```python
from build123d import *

# Parameters (mm, degrees)
EXTRUDE_1_DEPTH     = 280
SKETCH_2_R          = 2.2
CUT_EXTRUDE_1_DEPTH = 280
SKETCH_3_R          = 2.2
CUT_EXTRUDE_2_DEPTH = 20
CUT_EXTRUDE_3_DEPTH = 59
EXTRUDE_3_DEPTH     = 20
SKETCH_6_W          = 4.4
SKETCH_6_H          = 18
CUT_EXTRUDE_4_DEPTH = 20


with BuildPart() as part:
    # 草图1 → 凸台-拉伸1 (new body)
    with BuildSketch(Plane(origin=(0, 0, 0), x_dir=(1, 0, 0), z_dir=(0, 1, 0))):
        Polygon((10, 0), (10, 10), (0, 10), (-10, 10), (-10, 0), (-10, -10), (0, -10), (10, -10), align=None)
        Polygon((9, 0), (9, 9), (0, 9), (-9, 9), (-9, 0), (-9, -9), (0, -9), (9, -9), align=None, mode=Mode.SUBTRACT)
    extrude(amount=-EXTRUDE_1_DEPTH)

    # 草图2 → 切除-拉伸1 (cut)
    with BuildSketch(Plane.XY.offset(10)):
        with Locations(Location((0, -40, 0), (0, 0, 180))):
            Circle(SKETCH_2_R)
        with Locations(Location((0, -80, 0), (0, 0, 180))):
            Circle(SKETCH_2_R)
        with Locations(Location((0, -120, 0), (0, 0, 180))):
            Circle(SKETCH_2_R)
        with Locations(Location((0, -180, 0), (0, 0, 180))):
            Circle(SKETCH_2_R)
        with Locations(Location((0, -220, 0), (0, 0, 180))):
            Circle(SKETCH_2_R)
        with Locations(Location((0, -260, 0), (0, 0, 180))):
            Circle(SKETCH_2_R)
    extrude(amount=-CUT_EXTRUDE_1_DEPTH, mode=Mode.SUBTRACT)

    # 草图3 → 切除-拉伸2 (cut)
    with BuildSketch(Plane(origin=(10, 0, 0), x_dir=(0, 0, -1), z_dir=(1, 0, 0))):
        with Locations((0, -60)):
            Circle(SKETCH_3_R)
        with Locations((0, -100)):
            Circle(SKETCH_3_R)
        with Locations((0, -150)):
            Circle(SKETCH_3_R)
        with Locations((0, -200)):
            Circle(SKETCH_3_R)
        with Locations((0, -240)):
            Circle(SKETCH_3_R)
    extrude(amount=-CUT_EXTRUDE_2_DEPTH, mode=Mode.SUBTRACT)

    # 草图4 → 切除-拉伸3 (cut)
    with BuildSketch(Plane.XY.offset(10)):
        Polygon((0, -220), (10, -220), (10, 0), (-10, 0), (-10, -220), align=None)
    extrude(amount=-CUT_EXTRUDE_3_DEPTH, mode=Mode.SUBTRACT)

    # 草图5 → 凸台-拉伸3 (add)
    with BuildSketch(Plane.XY.offset(10)):
        with BuildLine():
            Line((-2.2, -220), (2.2, -220))
            ThreePointArc((2.2, -220), (0, -222.2), (-2.2, -220))
        make_face()
    extrude(amount=-EXTRUDE_3_DEPTH)

    # 草图6 → 切除-拉伸4 (cut)
    with BuildSketch(Plane(origin=(0, -220, 0), x_dir=(1, 0, 0), z_dir=(0, 1, 0))):
        Rectangle(SKETCH_6_W, SKETCH_6_H)
    extrude(amount=-CUT_EXTRUDE_4_DEPTH, mode=Mode.SUBTRACT)


solid = part.part
```
Geometry check sheet. Reference: the model listing, model coordinates, mm. A direction names the side the tool comes from. Coordinates: 2 decimals unless noted, no trailing zeros. Order: outer loops, then holes, each group sorted by start corner. A loop starts at its lowest first (then second) coordinate and runs counter-clockwise, first axis right, second up. Notation, with made-up numbers: (7.25, 26.25) - (20.25, 26.25) arc R17 ccw to (20.25, 49.25) - close; hole circle Ø3 at (67, 49.5). An arc over 180 degrees is marked (long way). Answer as a JSON object with one key per item and string values. Group by question number.
Item 1: Sectioned sample at C-C, the plane x = -5.25. Record the cut outline in (y, z), and give its area (3 significant figures).
Item 2: Draft check along Z on faces 1 (the face through (0.477, -257.852, -9.493)), 2 (the face through (9.507, -242.148, 0.477)), 3 (the face through (0, -250, 10)), 4 (the face through (0, -250, -10)). Enter one of: +Z half, -Z half, draft (parallel to the pull), parting line (faces both ways), or undercut.
Item 3: Scan lines: probe 1 along X at (y, z) = (-266.5, 7.25); probe 2 along Y at (x, z) = (9.6, 0). Record each from-to range of solid material in increasing order.
Item 4: Depth check by flat-ended pin: pin 1 Ø4 at (y, z) = (-240, 0) entering from +X. Enter the tip coordinate at first touch or a pass-through.
Item 5: Tool access check on faces 5 (the face through (0, -250, 9)), 6 (the face through (10, -250, 0)). Record the directions out of +Z, -Z, +X, -X, +Y, -Y that give a thin tool (end or side, any length) a straight path to the whole face; none if there is none.
Item 6: Sectioned sample at A-A, the plane z = 0. Record the cut outline in (x, y), and give its area (3 significant figures).
Item 7: Sectioned sample at D-D, the plane y = -248. Record the cut outline in (x, z), and give its area (3 significant figures).
Item 8: Sectioned sample at B-B, the plane y = -240. Record the cut outline in (x, z).
Resolved:
{
 "1": {"outline": "(-280, -10) - (-220, -10) - (-220, -9) - (-280, -9) - close; (-280, 9) - (-220, 9) - (-220, 10) - (-280, 10) - close", "area": "120 mm^2"},
 "2": {"face 1": "draft", "face 2": "undercut", "face 3": "+Z half", "face 4": "-Z half"},
 "3": {"probe 1": "-10 to -9, 9 to 10", "probe 2": "-280 to -242.2, -237.8 to -220"},
 "4": {"pin 1": "through"},
 "5": {"face 5": "+Y, -Y", "face 6": "+Z, -Z, +X, +Y, -Y"},
 "6": {"outline": "(-10, -280) - (-9, -280) - (-9, -242.2) - (-10, -242.2) - close; (-10, -237.8) - (-9, -237.8) - (-9, -220) - (-10, -220) - close; (9, -280) - (10, -280) - (10, -242.2) - (9, -242.2) - close; (9, -237.8) - (10, -237.8) - (10, -220) - (9, -220) - close", "area": "111 mm^2"},
 "7": {"outline": "(-10, -10) - (10, -10) - (10, 10) - (-10, 10) - close; hole (-9, -9) - (9, -9) - (9, 9) - (-9, 9) - close", "area": "76.0 mm^2"},
 "8": {"outline": "(-10, -10) - (10, -10) - (10, -2.2) - (9, -2.2) - (9, -9) - (-9, -9) - (-9, -2.2) - (-10, -2.2) - close; (-10, 2.2) - (-9, 2.2) - (-9, 9) - (9, 9) - (9, 2.2) - (10, 2.2) - (10, 10) - (-10, 10) - close"}
}
